Check sheet for the drawn part. Datum: minimum x, y, z corner. Units: mm. A direction names the side the tool comes from. Coordinates: 2 decimals unless noted, no trailing zeros. Loops run counter-clockwise (first coordinate to the right, second up) from the corner with the lowest first, then second, coordinate; pieces in that order, holes last.
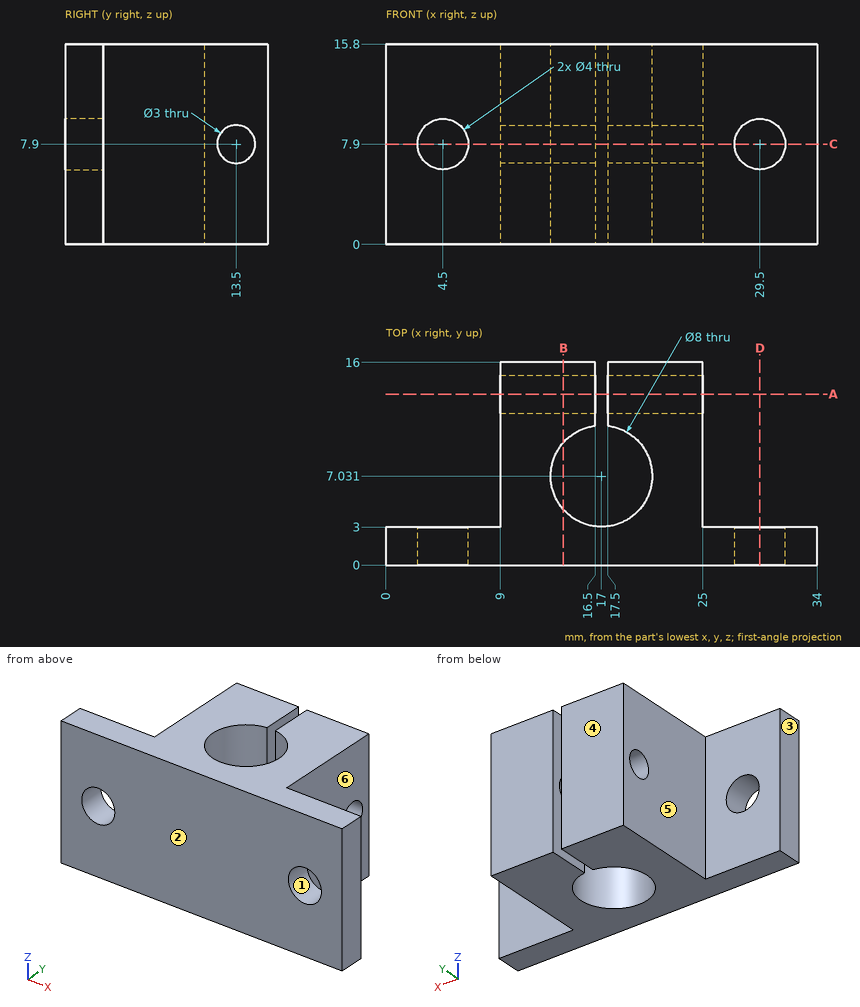
1) Section check B-B on x = 14. Enter the section's corners in (y, z) (1 decimal).
Answer sheet:
outline: (0, 0) - (4.4, 0) - (4.4, 15.8) - (0, 15.8) - close; (9.7, 0) - (16, 0) - (16, 15.8) - (9.7, 15.8) - close; hole circle Ø3 at (13.5, 7.9)
2) Section check D-D on x = 29.5. Enter the section's corners in (y, z), plus the area to 3 significant figures.
Answer sheet:
outline: (0, 0) - (3, 0) - (3, 5.9) - (0, 5.9) - close; (0, 9.9) - (3, 9.9) - (3, 15.8) - (0, 15.8) - close
area: 35.4 mm2
3) Section check A-A on y = 13.5. Enter the section's corners in (x, z), plus the area to 3 significant figures.
Answer sheet:
outline: (9, 0) - (16.5, 0) - (16.5, 6.4) - (9, 6.4) - close; (9, 9.4) - (16.5, 9.4) - (16.5, 15.8) - (9, 15.8) - close; (17.5, 0) - (25, 0) - (25, 6.4) - (17.5, 6.4) - close; (17.5, 9.4) - (25, 9.4) - (25, 15.8) - (17.5, 15.8) - close
area: 192 mm2
4) Depth check by flat-ended pin: pin 1 (4 mm diameter, centred on y = 13.5, z = 7.9, fed in from +X); pin 2 (2.5 mm diameter, centred on x = 3.5, z = 8.5, fed in from +Y); pin 3 (5 mm diameter, centred on y = 7.5, z = 12, fed in from -X). Enter the tip coordinate at first touch or a pass-through.
Answer sheet:
pin 1: stops at x = 25
pin 2: stops at y = 3
pin 3: stops at x = 9
5) Scan lines: line 1 (X direction, y = 1.3, z = 7.9); line 2 (X direction, y = 14.75, z = 14); line 3 (Y direction, x = 20.25, z = 7.9) (1 decimal). Record each from-to range of solid material in increasing order.
Answer sheet:
line 1: x = 0 to 2.5, 6.5 to 27.5, 31.5 to 34
line 2: x = 9 to 16.5, 17.5 to 25
line 3: y = 0 to 4.7, 9.4 to 12, 15 to 16
6) Mould release check, pull along X, two halves, no side actions. Record for the marked faces 1, 2 and 3: +X half, -X half, draft (parallel to the pull), parting line (faces both ways), or undercut.
Answer sheet:
face 1: undercut
face 2: draft
face 3: -X half
7) Section check C-C on z = 7.9. Enter the section's corners in (x, y), plus the area to 3 significant figures.
Answer sheet:
outline: (0, 0) - (2.5, 0) - (2.5, 3) - (0, 3) - close; (6.5, 0) - (27.5, 0) - (27.5, 3) - (25, 3) - (25, 12) - (17.5, 12) - (17.5, 11) arc R4 cw (long way) to (16.5, 11) - (16.5, 12) - (9, 12) - (9, 3) - (6.5, 3) - close; (9, 15) - (16.5, 15) - (16.5, 16) - (9, 16) - close; (17.5, 15) - (25, 15) - (25, 16) - (17.5, 16) - close; (31.5, 0) - (34, 0) - (34, 3) - (31.5, 3) - close
area: 186 mm2
8) Set-up check for the marked faces 4, 5 and 6: record each of +Z, -Z, +X, -X, +Y, -Y from which the full face is reachable in a straight line by a thin tool's end or side.
Answer sheet:
face 4: +Z, -Z, +X, -X, +Y
face 5: +Z, -Z, -X, +Y
face 6: +Z, -Z, +X, +Y
